Work out the finished part from the listing and answer in its coordinate system (mm). Face numbers are marked on the shaded views. A direction names the side the tool comes from. Give positions to 0.01 mm unless a question says otherwise; leave off trailing zeros. Write each loop counter-clockwise with the first axis right and the second up, starting at its lowest first coordinate (ties: lowest second). Pieces come first, ordered by that corner, then holes. Notation, with made-up numbers: (20.5, 27.25) -> (61.5, 27.25) arc R13 ccw to (61.5, 31.25) -> close; hole circle Ø4 at (45, 11.25). An arc over 180 degrees is marked (long way). Use a Markdown table: item, result. Add a question column.
Q1. For a pull along X with two mould halves and no side action, classify the marked faces 6, 7 and 8 as pulls with the +X half, pulls with the -X half, needs draft (parallel to the pull), parting line crosses it, or undercut.
Q2. Section A-A, the plane z = 0 is taken. State how many separate pieces and enclosed holes the cut face has, plus the area to 3 significant figures.
Q3. Section D-D, the plane y = 10 is taken. Give the vertices of the cut face in (x, z).
Q4. For the marked faces 1, 2, 3, 4 and 5, determine the directions among +Z, -Z, +X, -X, +Y, -Y from which every point of the face is accessible in a straight line to the end or side of a thin tool.
Q5. Each of these flat-tipped pins is pushed along its axis until it touches: pin 1 Ø11.5 at (x, z) = (0, -22.5) entering from +Y; pin 2 Ø16 at (x, z) = (-22.5, 0) entering from -Y; pin 3 Ø8 at (x, z) = (-15.91, -15.91) entering from +Y; pin 4 Ø1 at (x, y) = (26.5, -3.5) entering from +Z. Where does it stop, or does it pass through?
Q6. Consider line 1 (X direction, y = -0.5, z = 13.5); line 2 (X direction, y = -11, z = 8); line 3 (X direction, y = -9, z = 13). Determine where each line is inside the solid, lowest interval first.
from build123d import *

# Parameters (mm, degrees)
F2_R     = 10
F3_DEPTH = 40
F6_R     = 5
F7_DEPTH = 25


with BuildPart() as f1:
    # F0 (on Right) → F1 (revolve)
    with BuildSketch(Plane.YZ):
        Polygon((-20, 50), (-20, 0), (20, 0), (20, 50), (13, 50), (6, 37.5), (0, 37.5), (-6, 37.5), (-13, 50), align=None)
    revolve(axis=Axis((0, 0, 0), (0, 1, 0)))

    # F2 (on face) → F3 (cut)
    with BuildSketch(Plane.XZ.offset(20)):
        Circle(F2_R)
    extrude(amount=-F3_DEPTH, mode=Mode.SUBTRACT)

    # F4 (on Right) → F5 (revolve, cut)
    with BuildSketch(Plane.YZ):
        Polygon((-15, -10), (-20, -10), (-20, -32), (-6, -28), (-6, -17), (-15, -17), align=None)
        Polygon((15, -17), (6, -17), (6, -28), (20, -32), (20, -10), (15, -10), align=None)
    revolve(axis=Axis((0, -10, 0), (0, -1, 0)), mode=Mode.SUBTRACT)

    # F6 (on face) → F7 (cut)
    with BuildSketch(Plane.XZ.offset(6)):
        with Locations((-15.909903, 15.909903)):
            Circle(F6_R)
        with Locations((0, 22.5)):
            Circle(F6_R)
        with Locations((15.909903, 15.909903)):
            Circle(F6_R)
        with Locations((-22.5, 0)):
            Circle(F6_R)
        with Locations((-15.909903, -15.909903)):
            Circle(F6_R)
        with Locations((0, -22.5)):
            Circle(F6_R)
        with Locations((15.909903, -15.909903)):
            Circle(F6_R)
        with Locations((22.5, 0)):
            Circle(F6_R)
    extrude(amount=-F7_DEPTH, mode=Mode.SUBTRACT)


solid = f1.part
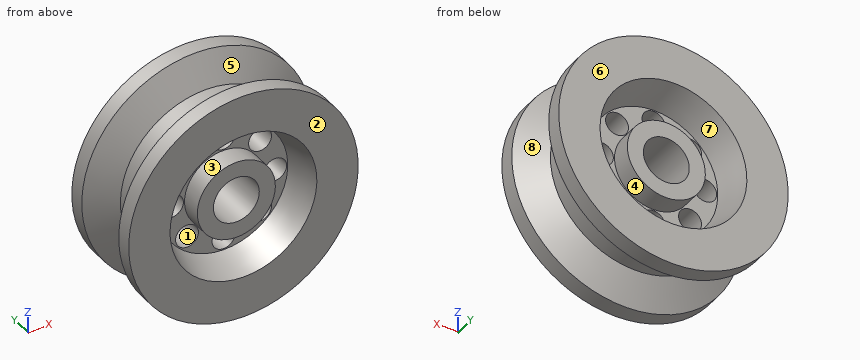
Result set:
| question | item | result |
|---|---|---|
| 1 | face 6 | needs draft |
| 1 | face 7 | undercut |
| 1 | face 8 | parting line crosses it |
| 2 | separate pieces | 4 |
| 2 | enclosed holes | 0 |
| 2 | area | 1,620 mm2 |
| 3 | outline | circle Ø89.29 at (0, 0); circle Ø34 at (0, 0); hole circle Ø58.29 at (0, 0); hole circle Ø20 at (0, 0) |
| 4 | face 1 | +Y, -Y |
| 4 | face 2 | +Z, -Z, +X, -X, -Y |
| 4 | face 3 | -Y |
| 4 | face 4 | +Y |
| 4 | face 5 | none |
| 5 | pin 1 | stops at y = 15 |
| 5 | pin 2 | stops at y = -15 |
| 5 | pin 3 | passes through |
| 5 | pin 4 | stops at z = 27.02 |
| 6 | line 1 | x = -34.99 to -20.29, -11.53 to 11.53, 20.29 to 34.99 |
| 6 | line 2 | x = -45.73 to -28.32, -15 to -6, 6 to 15, 28.32 to 45.73 |
| 6 | line 3 | x = -40.84 to -25.76, -10.95 to 10.95, 25.76 to 40.84 |
